```python
from build123d import *

# Parameters (mm, degrees)
BOSS_EXTRUDE1_DEPTH                   = 12.7
TAP_DRILL_FOR_M5X0_8_TAP1_D           = 4.2
TAP_DRILL_FOR_M5X0_8_TAP1_CSINK_D     = 4.25
TAP_DRILL_FOR_M5X0_8_TAP1_CSINK_ANGLE = 90
M6_CLEARANCE_HOLE1_D                  = 6.4
M6_CLEARANCE_HOLE1_CSINK_D            = 6.65
M6_CLEARANCE_HOLE1_CSINK_ANGLE        = 90
FILLET1_R                             = 1


with BuildPart() as part:
    # Sketch1 → Boss-Extrude1 (new body)
    with BuildSketch(Plane.XY):
        Polygon((-26, 0), (26, 0), (26, 6), (26, 22), (7.5, 22), (-7.5, 22), (-26, 22), (-26, 6), align=None)
    extrude(amount=-BOSS_EXTRUDE1_DEPTH)

    # Tap Drill for M5x0.8 Tap1 (through all)
    with Locations(Plane(origin=(0, 11, 0), x_dir=(1, 0, 0), z_dir=(0, 0, 1))):
        with Locations((0, 0)):
            CounterSinkHole(TAP_DRILL_FOR_M5X0_8_TAP1_D / 2, TAP_DRILL_FOR_M5X0_8_TAP1_CSINK_D / 2, counter_sink_angle=TAP_DRILL_FOR_M5X0_8_TAP1_CSINK_ANGLE)

    # M6 Clearance Hole1 (through all)
    with Locations(Plane(origin=(-20, 0, -6.35), x_dir=(-1, 0, 0), z_dir=(0, -1, 0))):
        with Locations((0, 0), (-40, 0)):
            CounterSinkHole(M6_CLEARANCE_HOLE1_D / 2, M6_CLEARANCE_HOLE1_CSINK_D / 2, counter_sink_angle=M6_CLEARANCE_HOLE1_CSINK_ANGLE)

    # Fillet1
    fillet1_edges = [part.edges().sort_by_distance(p)[0] for p in [
        (-26, 22, -6.35),
        (26, 22, -6.35),
    ]]
    fillet(fillet1_edges, radius=FILLET1_R)


solid = part.part
```
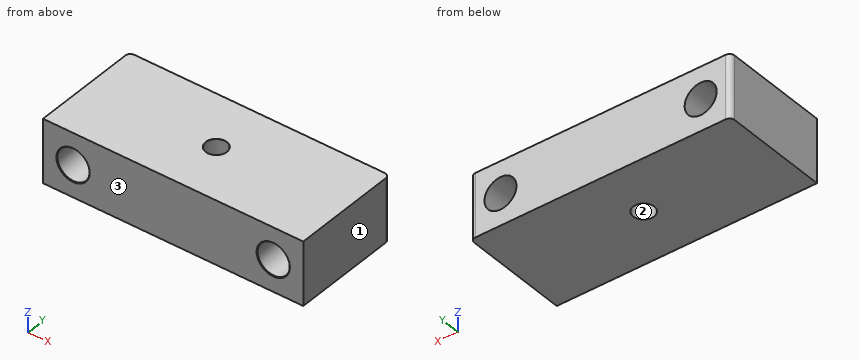
CAD build for the part. Positions are in the model's coordinates, mm. Face numbers are marked on the shaded views. Coordinates: 2 decimals unless noted, no trailing zeros. Write each loop counter-clockwise with the first axis right and the second up, starting at its lowest first coordinate (ties: lowest second). Pieces come first, ordered by that corner, then holes. Notation, with made-up numbers: (6.25, 19.5) -> (15.25, 19.5) arc R32 ccw to (15.25, 55.5) -> close; hole circle Ø5 at (70, 35). An arc over 180 degrees is marked (long way). Return JSON: item names as keys, results as strings. Group by question number.
Q1. Pull direction Y, two halves, no side cores. Call the marked faces 1, 2 and 3: released by +Y, released by -Y, zero draft, split by the parting line, or undercut.
Q2. Cut at A-A, the plane y = 11. Give the cut face in (x, z) (3 decimals).
Q3. Cut at D-D, the plane x = 0. Give the cut face in (y, z) (3 decimals), then the cut area to 3 significant figures.
Q4. Cut at B-B, the plane z = -6.35. Give the cut face in (x, y) (3 decimals), then the cut area to 3 significant figures.
Q5. Drill centre lines: line 1 (X direction, y = 19.25, z = -5.25) (3 decimals); line 2 (Z direction, x = 20, y = 5.5); line 3 (X direction, y = 7.75, z = -3.5). Where is each one in solid material? Low to high.
Q6. Cut at C-C, the plane x = 20. Give the cut face in (y, z) (3 decimals).
Returned:
{
 "1": {"face 1": "zero draft", "face 2": "undercut", "face 3": "released by -Y"},
 "2": {"outline": "(-26, -12.7) -> (-2.1, -12.7) -> (-2.1, -0.025) -> (-2.125, 0) -> (-26, 0) -> close; (2.1, -12.7) -> (26, -12.7) -> (26, 0) -> (2.125, 0) -> (2.1, -0.025) -> close; hole circle Ø6.4 at (-20, -6.35); hole circle Ø6.4 at (20, -6.35)"},
 "3": {"outline": "(0, -12.7) -> (8.9, -12.7) -> (8.9, -0.025) -> (8.875, 0) -> (0, 0) -> close; (13.1, -12.7) -> (22, -12.7) -> (22, 0) -> (13.125, 0) -> (13.1, -0.025) -> close", "area": "226 mm2"},
 "4": {"outline": "(-26, 0) -> (-23.325, 0) -> (-23.2, 0.125) -> (-23.2, 22) -> (-25, 22) arc R1 ccw to (-26, 21) -> close; (-16.8, 0.125) -> (-16.675, 0) -> (16.675, 0) -> (16.8, 0.125) -> (16.8, 22) -> (-16.8, 22) -> close; (23.2, 0.125) -> (23.325, 0) -> (26, 0) -> (26, 21) arc R1 ccw to (25, 22) -> (23.2, 22) -> close; hole circle Ø4.2 at (0, 11)", "area": "848 mm2"},
 "5": {"line 1": "x = -26 to -23.005, -16.995 to 16.995, 23.005 to 26", "line 2": "z = -12.7 to -9.55, -3.15 to 0", "line 3": "x = -26 to -21.46, -18.54 to 18.54, 21.46 to 26"},
 "6": {"outline": "(0, -12.7) -> (22, -12.7) -> (22, -9.55) -> (0.125, -9.55) -> (0, -9.675) -> close; (0, -3.025) -> (0.125, -3.15) -> (22, -3.15) -> (22, 0) -> (0, 0) -> close"}
}
